Part print with two shaded views. Sizes in mm from the minimum x, y, z corner. Give positions to 0.01 mm unless a question says otherwise; leave off trailing zeros. Write each loop counter-clockwise with the first axis right and the second up, starting at its lowest first coordinate (ties: lowest second). Pieces come first, ordered by that corner, then holes. Notation, with made-up numbers: M 57.5,41.25 L 106.5,41.25 A28 ccw 106.5,71.25 Z; hole C 31.25,-1.5 d7. An arc over 180 degrees is marked long. Return JSON: item names as keys, results as strings. Group by question number.
Q1. Wall check: probe 1 along X at (y, z) = (1.5, 35.56) (3 decimals); probe 2 along Z at (x, y) = (22, 1.5); probe 3 along Z at (x, y) = (256.5, 3.5). Give the ranges that are in metal, low to high.
Q2. Flat gauge pin, fed straight in: pin 1 Ø11.5 at (x, z) = (257.175, 264.16) entering from -Y. Where does the tip first touch, or does it go through?
Q3. Band-saw the part on B-B, the plane z = 38.5. Give the cut face in (x, y).
Q4. Band-saw the part on A-A, the plane z = 264.16. Give the cut face in (x, y) (3 decimals), then the cut area to 3 significant figures.
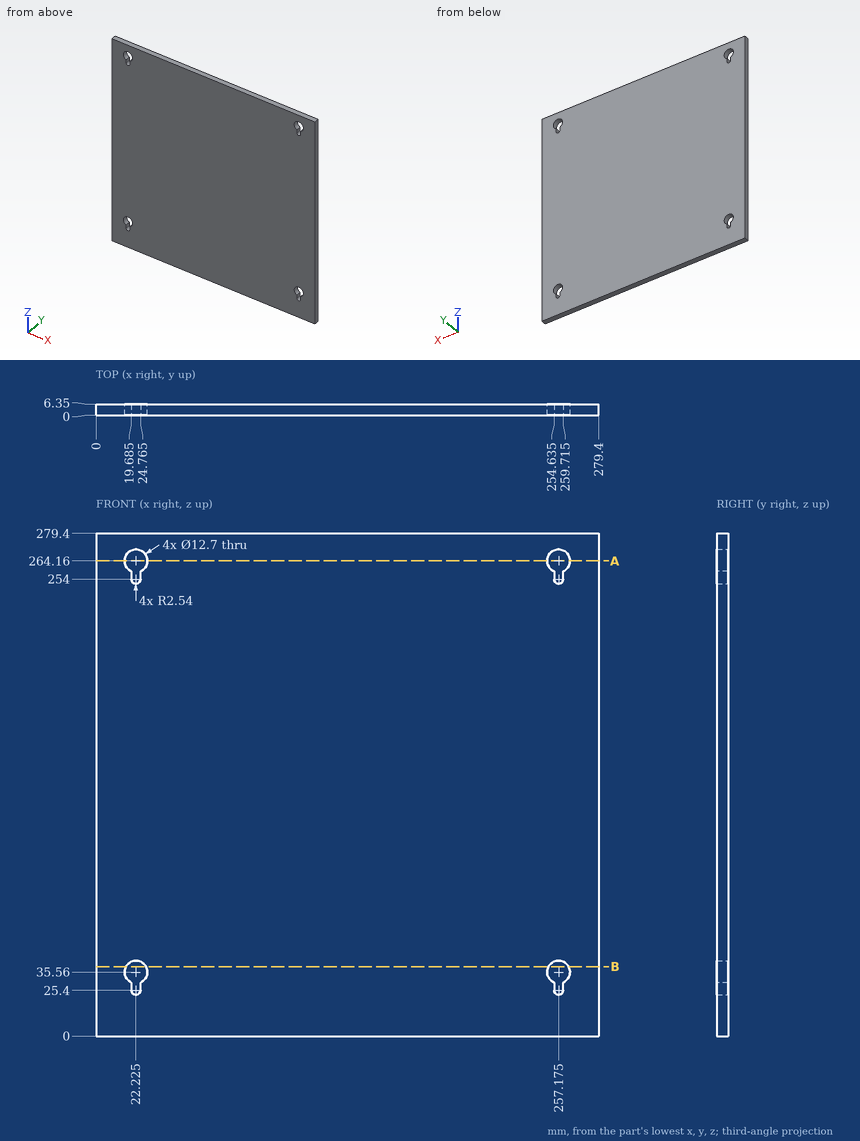
From the geometry:
{
 "1": {"probe 1": "x = 0 to 15.875, 28.575 to 250.825, 263.525 to 279.4", "probe 2": "z = 0 to 22.87, 41.91 to 251.47, 270.51 to 279.4", "probe 3": "z = 0 to 22.95, 41.87 to 251.55, 270.47 to 279.4"},
 "2": {"pin 1": "passes through"},
 "3": {"outline": "M 0,0 L 16.6,0 L 16.6,6.35 L 0,6.35 Z; M 27.85,0 L 251.55,0 L 251.55,6.35 L 27.85,6.35 Z; M 262.8,0 L 279.4,0 L 279.4,6.35 L 262.8,6.35 Z"},
 "4": {"outline": "M 0,0 L 15.875,0 L 15.875,6.35 L 0,6.35 Z; M 28.575,0 L 250.825,0 L 250.825,6.35 L 28.575,6.35 Z; M 263.525,0 L 279.4,0 L 279.4,6.35 L 263.525,6.35 Z", "area": "1,610 mm^2"}
}
